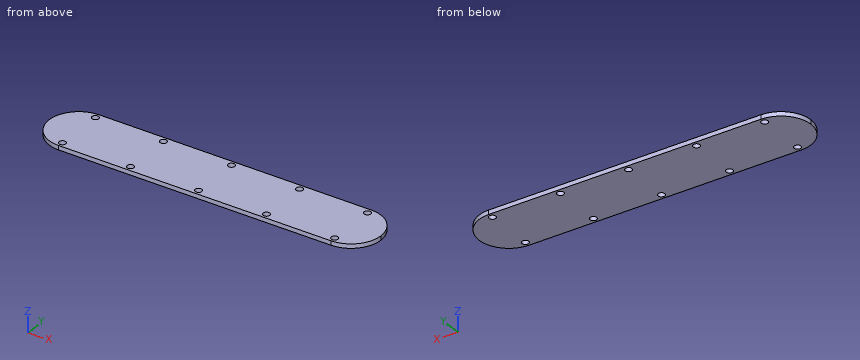
from build123d import *

# Parameters (mm, degrees)
SKETCH1_W                    = 247.65
SKETCH1_H                    = 44.45
BOSS_EXTRUDE1_DEPTH          = 3.175
CUT_EXTRUDE1_DEPTH           = 126.84379951
F_10_0_1935_DIAMETER_HOLE1_D = 4.999999906


with BuildPart() as part:
    # Sketch1 → Boss-Extrude1 (new body)
    with BuildSketch(Plane.XY):
        Rectangle(SKETCH1_W, SKETCH1_H)
    extrude(amount=BOSS_EXTRUDE1_DEPTH)

    # Sketch2 → Cut-Extrude1 (cut, through all)
    with BuildSketch(Plane.XY.offset(3.175)):
        with BuildLine():
            Line((-123.825, 22.225), (-123.825, 5e-09))
            ThreePointArc((-123.825, 5e-09), (-117.31544821, 15.715448214), (-101.6, 22.225))
            Line((-101.6, 22.225), (-123.825, 22.225))
        make_face()
        with BuildLine():
            Line((-123.825, -22.225), (-101.6, -22.225))
            ThreePointArc((-101.6, -22.225), (-117.315448214, -15.71544821), (-123.825, 5e-09))
            Line((-123.825, 5e-09), (-123.825, -22.225))
        make_face()
        with BuildLine():
            ThreePointArc((123.825, -6.4e-08), (117.315448189, -15.715448235), (101.6, -22.225))
            Line((101.6, -22.225), (123.825, -22.225))
            Line((123.825, -22.225), (123.825, -6.4e-08))
        make_face()
        with BuildLine():
            ThreePointArc((101.6, 22.225), (117.315448235, 15.715448189), (123.825, -6.4e-08))
            Line((123.825, -6.4e-08), (123.825, 22.225))
            Line((123.825, 22.225), (101.6, 22.225))
        make_face()
    extrude(amount=-CUT_EXTRUDE1_DEPTH, mode=Mode.SUBTRACT)

    # #10 (0.1935) Diameter Hole1 (through all)
    with Locations(Plane.XY.offset(3.175)):
        with Locations((-101.6, 18.161), (-50.8, 18.161), (0, 18.161), (50.8, 18.161), (101.6, 18.161), (101.6, -18.161), (50.8, -18.161), (0, -18.161), (-50.8, -18.161), (-101.6, -18.161)):
            Hole(F_10_0_1935_DIAMETER_HOLE1_D / 2)


solid = part.part
Work out the finished part from the listing and answer in its coordinate system (mm). Give positions to 0.01 mm unless a question says otherwise; leave off trailing zeros. Order: outer loops, then holes, each group sorted by start corner. A loop starts at its lowest first (then second) coordinate and runs counter-clockwise, first axis right, second up. Notation, with made-up numbers: (-24.5, 31.5) - (16.5, 31.5) arc R13 ccw to (16.5, 36.5) - close; hole circle Ø10 at (37.25, 0.25). An arc over 180 degrees is marked (long way). Answer as CSV lines item,"result". Start each with the question number.
Q1. The part is cut by section D-D (y = -10). Write down the section's boundary in (x, z) (3 decimals).
Q2. Find the intervals of material crossed by L1, parallel to Y at x = -101.6, z = 2.45 (3 decimals); L2, parallel to X at y = 16, z = 0.35; L3, parallel to X at y = -17.5, z = 1.2, in increasing order. Write a range as [from, to].
Q3. The part is cut by section B-B (z = 1.7). Give the number of separate pieces and of enclosed holes in the cut face, then the cut area to 3 significant figures.
Q4. The part is cut by section A-A (x = -50.8). Write down the section's boundary in (y, z) (3 decimals), then the cut area to 3 significant figures.
Q5. Given pin 1 Ø6.5 at (x, y) = (-50.8, -18.161) entering from -Z; pin 2 Ø4.5 at (x, y) = (50.8, 18.161) entering from -Z, each flat-ended and moving along its own axis, determine where each tip first touches the part or whether it passes through.
Q6. The part is cut by section C-C (y = 9). Write down the section's boundary in (x, z) (3 decimals), then the cut area to 3 significant figures.
Check result:
1,outline,"(-121.448, 0) - (121.448, 0) - (121.448, 3.175) - (-121.448, 3.175) - close"
2,L1,"y = [-22.225, -20.661], [-15.661, 15.661], [20.661, 22.225]"
2,L2,"x = [-117.03, -102.86], [-100.34, -52.06], [-49.54, -1.26], [1.26, 49.54], [52.06, 100.34], [102.86, 117.03]"
2,L3,"x = [-115.3, -104.01], [-99.19, -53.21], [-48.39, -2.41], [2.41, 48.39], [53.21, 99.19], [104.01, 115.3]"
3,separate pieces,"1"
3,enclosed holes,"10"
3,area,"10,400 mm²"
4,outline,"(-22.225, 0) - (-20.661, 0) - (-20.661, 3.175) - (-22.225, 3.175) - close; (-15.661, 0) - (15.661, 0) - (15.661, 3.175) - (-15.661, 3.175) - close; (20.661, 0) - (22.225, 0) - (22.225, 3.175) - (20.661, 3.175) - close"
4,area,"109 mm²"
5,pin 1,"stops at z = 0"
5,pin 2,"passes through"
6,outline,"(-121.921, 0) - (121.921, 0) - (121.921, 3.175) - (-121.921, 3.175) - close"
6,area,"774 mm²"
